Build history of the part. All positions in model axes, mm. Face numbers are marked on the shaded views. A direction names the side the tool comes from. Coordinates: 2 decimals unless noted, no trailing zeros. Write each loop counter-clockwise with the first axis right and the second up, starting at its lowest first coordinate (ties: lowest second). Pieces come first, ordered by that corner, then holes.
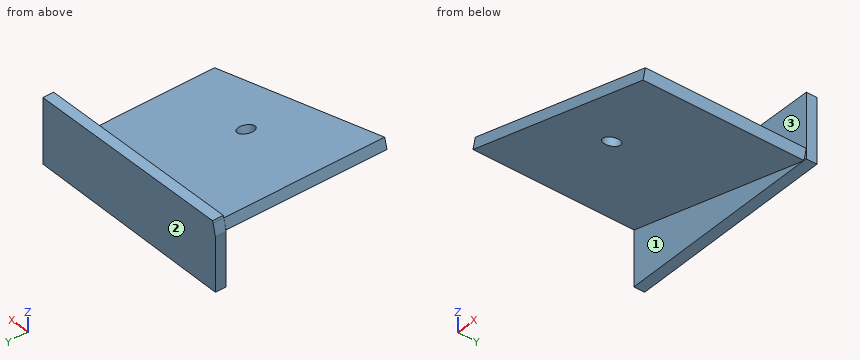
```python
from build123d import *

# Parameters (mm, degrees)
BOSS_EXTRUDE1_DEPTH = 4
BOSS_EXTRUDE3_DEPTH = 60
SKETCH8_R           = 3
CUT_EXTRUDE2_DEPTH  = 79
BOSS_EXTRUDE5_START = -4
BOSS_EXTRUDE5_DEPTH = 4
CUT_EXTRUDE3_DEPTH  = 4
SKETCH14_W          = 38.062003052
SKETCH14_H          = 100
CUT_EXTRUDE4_DEPTH  = 4
CUT_EXTRUDE5_DEPTH  = 10
SKETCH16_W          = 78.309342284
SKETCH16_H          = 4
BOSS_EXTRUDE6_DEPTH = 10
CUT_EXTRUDE6_DEPTH  = 10


with BuildPart() as part:
    # Sketch1 → Boss-Extrude1 (new body)
    with BuildSketch(Plane(origin=(0, 0, 0), x_dir=(1, 0, 0), z_dir=(0, 1, 0))):
        with BuildLine():
            Line((0, 0), (-80, 0))
            ThreePointArc((-80, 0), (-79.31558891, -10.442095378), (-77.274066103, -20.705523608))
            Line((-77.274066103, -20.705523608), (0, 0))
        make_face()
    extrude(amount=BOSS_EXTRUDE1_DEPTH)

    # Sketch7 → Boss-Extrude3 (add)
    with BuildSketch(Plane.XZ):
        Polygon((0, 0), (-77.274066103, 20.705523608), (-78.309342284, 16.841820303), (-1.03527618, -3.863703305), align=None)
    extrude(amount=BOSS_EXTRUDE3_DEPTH)

    # Sketch8 → Cut-Extrude2 (cut)
    with BuildSketch(Plane(origin=(-1.03527618, 0, -3.863703305), x_dir=(-0.9659258262890682, 0, 0.25881904510252124), z_dir=(-0.25881904510252124, 0, -0.9659258262890682))):
        with Locations((40, -40)):
            Circle(SKETCH8_R)
    extrude(amount=-CUT_EXTRUDE2_DEPTH, mode=Mode.SUBTRACT)

    # Sketch11 → Boss-Extrude5 (add)
    with BuildSketch(Plane(origin=(0, 4, 0), x_dir=(1, 0, 0), z_dir=(0, 1, 0)).offset(BOSS_EXTRUDE5_START)):
        with BuildLine():
            Line((0, 0), (-77.274066103, -20.705523608))
            ThreePointArc((-77.274066103, -20.705523608), (-48.700914321, -63.468267223), (0, -80))
            Line((0, -80), (0, 0))
        make_face()
    extrude(amount=BOSS_EXTRUDE5_DEPTH)

    # Sketch12 → Cut-Extrude3 (cut)
    with BuildSketch(Plane.XZ):
        Polygon((-68.830314461, 40.772390306), (32.565775989, 40.772390306), (32.565775989, 109.047215686), (-78.543674294, 109.047215686), align=None)
    extrude(amount=-CUT_EXTRUDE3_DEPTH, mode=Mode.SUBTRACT)

    # Sketch14 → Cut-Extrude4 (cut)
    with BuildSketch(Plane.XZ):
        with Locations((-97.34034381, -33.158179697)):
            Rectangle(SKETCH14_W, SKETCH14_H)
    extrude(amount=-CUT_EXTRUDE4_DEPTH, mode=Mode.SUBTRACT)

    # Sketch15 → Cut-Extrude5 (cut)
    with BuildSketch(Plane(origin=(0, 0, 0), x_dir=(-1, 0, 0), z_dir=(0, -1, 0))):
        Polygon((81.89924148, -21.519578019), (0, -20.386195153), (0, -64.251910572), (85.684715325, -64.251910572), align=None)
    extrude(amount=-CUT_EXTRUDE5_DEPTH, mode=Mode.SUBTRACT)

    # Sketch16 → Boss-Extrude6 (add)
    with BuildSketch(Plane(origin=(0, 0, 0), x_dir=(-1, 0, 0), z_dir=(0, 0, -1))):
        with Locations((39.154671142, 2)):
            Rectangle(SKETCH16_W, SKETCH16_H)
    extrude(amount=BOSS_EXTRUDE6_DEPTH)

    # Sketch17 → Cut-Extrude6 (cut)
    with BuildSketch(Plane(origin=(0, 0, 0), x_dir=(-1, 0, 0), z_dir=(0, -1, 0))):
        Polygon((1.203546953, 3.818615287), (78.309342284, 3.818615287), (78.309342284, 14.954407394), (-14.190924513, 13.37318069), (-14.190924513, 3.818615287), align=None)
    extrude(amount=-CUT_EXTRUDE6_DEPTH, mode=Mode.SUBTRACT)


solid = part.part
```
1. Saw through at A-A on y = -39. List the corners of the cut face in (x, z).
Computed values:
outline: (-78.31, 16.84) - (-42.4, 7.22) - (-41.37, 11.08) - (-77.27, 20.71) - close; (-36.94, 5.76) - (-1.04, -3.86) - (0, 0) - (-35.9, 9.62) - close
2. Flat gauge pins, fed straight in: pin 1 (4 mm diameter, centred on x = -43.5, y = -44.5, fed in from +Z); pin 2 (4.5 mm diameter, centred on x = -40, y = 3, fed in from -Z); pin 3 (10 mm diameter, centred on x = -14, y = -31.5, fed in from +Z); pin 4 (4 mm diameter, centred on x = -19.5, z = 0.5, fed in from -Y). Where does each tip first touch, or does it go through?
Computed values:
pin 1: stops at z = 12.19
pin 2: stops at z = -3.82
pin 3: stops at z = 5.09
pin 4: stops at y = -60
3. 3-axis set-ups, long thin cutter, end or side, ignore diameter. For the marked faces 1, 2 and 3: which of +Z, -Z, +X, -X, +Y, -Y reach the whole face in a straight line?
Computed values:
face 1: -Z, -X, -Y
face 2: +Z, -Z, +X, -X, +Y
face 3: +Z, +X, -Y
4. Probe line 1 along Y through (x, z) = (-38, 9); line 2 along Y through (x, z) = (-12, 6.25); line 3 along Z through (x, y) = (-5.5, -26.5). List the from-to ranges inside material, lowest first.
Computed values:
line 1: y = -60 to -42.84, -37.16 to 4
line 2: y = 0 to 4
line 3: z = -2.67 to 1.47
5. Saw through at B-B on z = 1.5. List the corners of the cut face in (x, y), plus the area to 3 significant figures.
Computed values:
outline: (-78.31, 0) - (-21.05, 0) - (-21.05, -60) - (-5.6, -60) - (-5.6, 0) - (0, 0) - (0, 4) - (-78.31, 4) - close
area: 1,240 mm2
6. Saw through at C-C on x = -14.5. List the corners of the cut face in (y, z), plus the area to 3 significant figures.
Computed values:
outline: (-60, -0.26) - (0, -0.26) - (0, -3.82) - (4, -3.82) - (4, 20.59) - (0, 20.59) - (0, 3.89) - (-60, 3.89) - close
area: 346 mm2
